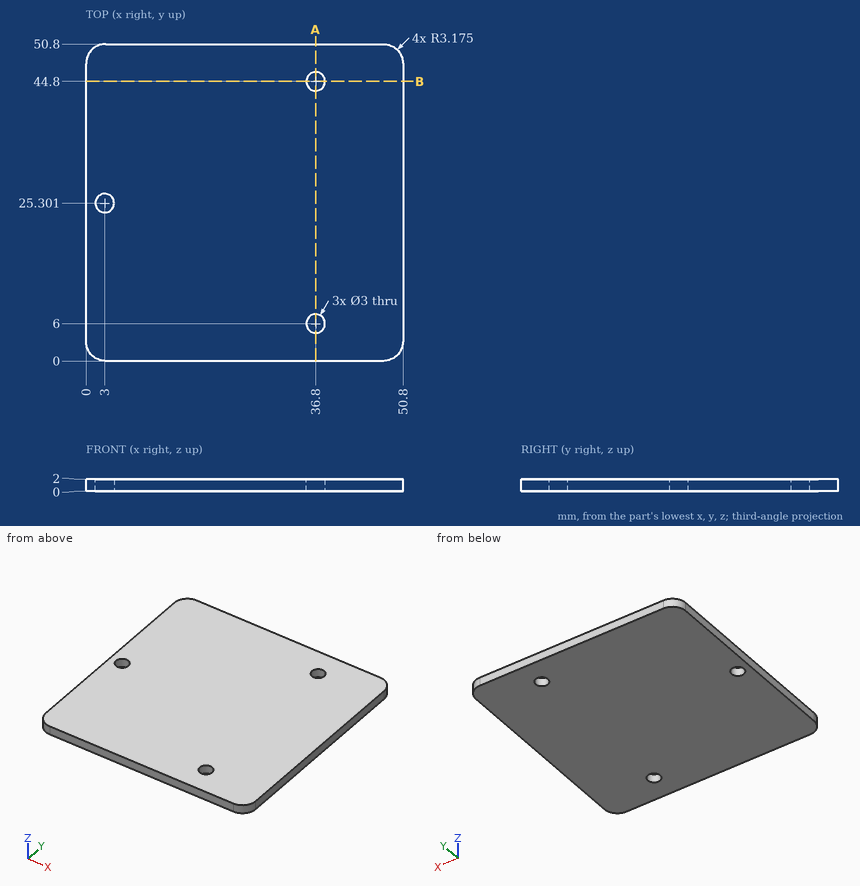
Can you work these out from the drawing? Everything is in mm from the part's minimum corner. Coordinates: 2 decimals unless noted, no trailing zeros. Write each loop counter-clockwise with the first axis right and the second up, starting at its lowest first coordinate (ties: lowest second). Pieces come first, ordered by that corner, then holes. Notation, with made-up numbers: (-12, 66) - (5, 66) arc R11 cw to (5, 70) - close; hole circle Ø11 at (-18, -1). An arc over 180 degrees is marked (long way). Use a Markdown table: item, result.
Q1. Imagine slicing it at B-B (y = 44.8). List the corners of the cut face in (x, z) for me.
Geometry check:
| item | result |
|---|---|
| outline | (0, 0) - (35.3, 0) - (35.3, 2) - (0, 2) - close; (38.3, 0) - (50.8, 0) - (50.8, 2) - (38.3, 2) - close |
Q2. I'm going to push a flat-ended pin straight in: pin 1 Ø2.5 at (x, y) = (36.8, 44.8) entering from -Z. Where does the tip first touch, or does it pass through?
Geometry check:
| item | result |
|---|---|
| pin 1 | passes through |
Q3. Imagine slicing it at A-A (x = 36.8). List the corners of the cut face in (y, z) for me.
Geometry check:
| item | result |
|---|---|
| outline | (0, 0) - (4.5, 0) - (4.5, 2) - (0, 2) - close; (7.5, 0) - (43.3, 0) - (43.3, 2) - (7.5, 2) - close; (46.3, 0) - (50.8, 0) - (50.8, 2) - (46.3, 2) - close |
Q4. Please list where these lines run through material, in increasing order: L1, parallel to Y at x = 36.8, z = 1.3; L2, parallel to X at y = 45, z = 0.2; L3, parallel to Y at x = 3, z = 0.65 (1 decimal).
Geometry check:
| item | result |
|---|---|
| L1 | y = 0 to 4.5, 7.5 to 43.3, 46.3 to 50.8 |
| L2 | x = 0 to 35.31, 38.29 to 50.8 |
| L3 | y = 0 to 23.8, 26.8 to 50.8 |
